Print and shaded views of the part. All mm, measured from the part's lowest x, y and z. A direction names the side the tool comes from. Coordinates: 2 decimals unless noted, no trailing zeros. Order: outer loops, then holes, each group sorted by start corner. A loop starts at its lowest first (then second) coordinate and runs counter-clockwise, first axis right, second up. Notation, with made-up numbers: (29, -9.5) -> (48, -9.5) arc R23 cw to (48, 22.5) -> close; hole circle Ø4 at (-31, -21). An arc over 180 degrees is marked (long way). Return JSON: item names as keys, results as strings. Group by question number.
1) Pull direction X, two halves, no side cores. Call the marked faces 3, 4 and 5: +X half, -X half, draft (parallel to the pull), parting line (faces both ways), or undercut.
2) Probe line 1 (X direction, y = 2, z = 5.3); line 2 (X direction, y = 3, z = 4.25); line 3 (Z direction, x = 5.5, y = 1.5) (3 decimals). List the from-to ranges inside material, lowest first.
3) Cut at A-A (x = 5.3). Write the cut outline in (y, z).
4) Cut at C-C (y = 4.75). Write the cut outline in (x, z), and give its area (3 significant figures).
5) Cut at B-B (z = 5.3). Write the cut outline in (x, y).
6) Which spindle directions (+Z, -Z, +X, -X, +Y, -Y) get a long thin tool onto all of the face, cutting with end or side? Do the marked faces 1 and 2. Say none if no direction does.
7) Flat gauge pins, fed straight in: pin 1 (1 mm diameter, centred on y = 3.5, z = 5.5, fed in from +X); pin 2 (4 mm diameter, centred on x = 8, y = 4.5, fed in from -Z); pin 3 (1 mm diameter, centred on x = 6.5, y = 3, fed in from -Z); pin 4 (2.5 mm diameter, centred on x = 5.3, z = 5.3, fed in from -Y). Where does each tip first touch, or does it go through?
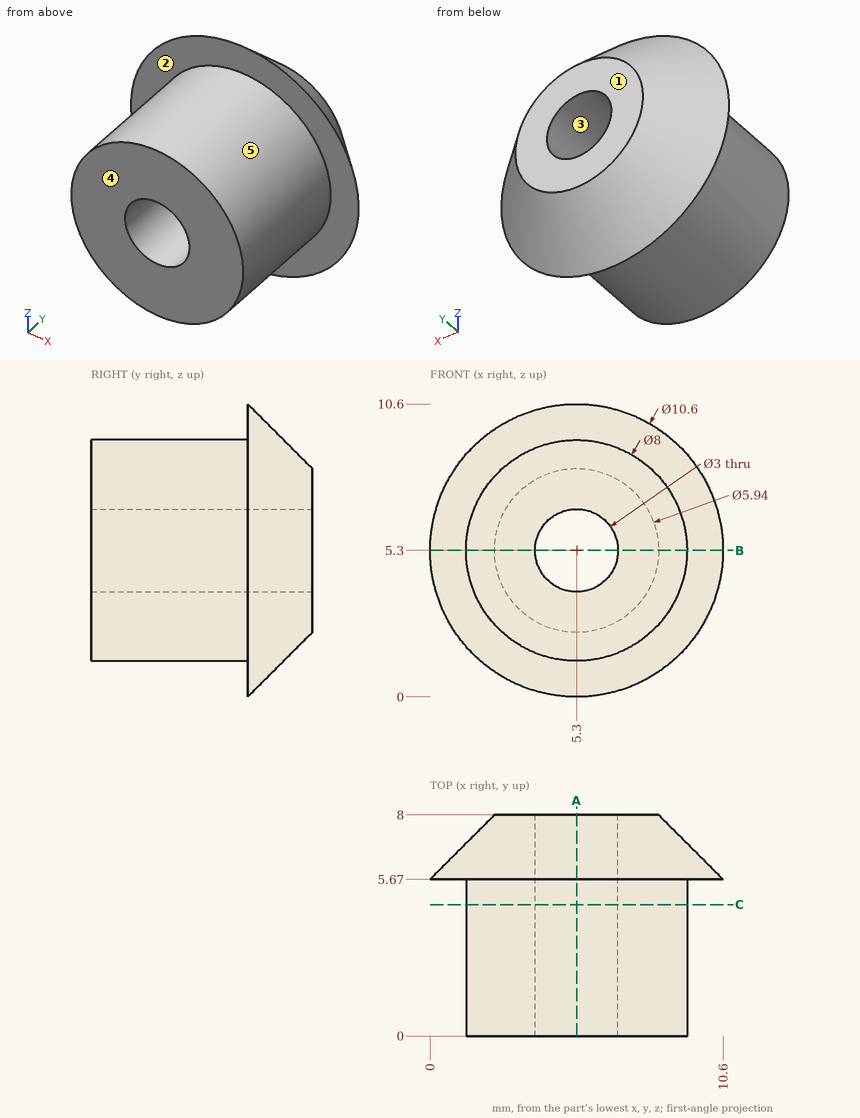
Answers below:
{
 "1": {"face 3": "undercut", "face 4": "draft", "face 5": "parting line"},
 "2": {"line 1": "x = 1.3 to 3.8, 6.8 to 9.3", "line 2": "x = 1.44 to 4.23, 6.37 to 9.16", "line 3": "z = 1.305 to 3.813, 6.787 to 9.295"},
 "3": {"outline": "(0, 1.3) -> (5.67, 1.3) -> (5.67, 0) -> (8, 2.33) -> (8, 3.8) -> (0, 3.8) -> close; (0, 6.8) -> (8, 6.8) -> (8, 8.27) -> (5.67, 10.6) -> (5.67, 9.3) -> (0, 9.3) -> close"},
 "4": {"outline": "circle Ø8 at (5.3, 5.3); hole circle Ø3 at (5.3, 5.3)", "area": "43.2 mm^2"},
 "5": {"outline": "(0, 5.67) -> (1.3, 5.67) -> (1.3, 0) -> (3.8, 0) -> (3.8, 8) -> (2.33, 8) -> close; (6.8, 0) -> (9.3, 0) -> (9.3, 5.67) -> (10.6, 5.67) -> (8.27, 8) -> (6.8, 8) -> close"},
 "6": {"face 1": "+Z, -Z, +X, -X, +Y", "face 2": "-Y"},
 "7": {"pin 1": "stops at x = 9.3", "pin 2": "stops at z = 0.11", "pin 3": "stops at z = 1.36", "pin 4": "passes through"}
}
